```python
from build123d import *

# Parameters (mm, degrees)
SKETCH1_W                     = 104.5
SKETCH1_H                     = 59.5
BOSS_EXTRUDE1_DEPTH           = 73.36
CBORE_FOR_M4_SHCS2_AT_2_COUNT = 2
CBORE_FOR_M4_SHCS2_AT_2_PITCH = 73
CBORE_FOR_M4_SHCS2_AT_3_COUNT = 2
CBORE_FOR_M4_SHCS2_AT_3_PITCH = 83.725742756
CBORE_FOR_M4_SHCS2_AT_4_COUNT = 2
CBORE_FOR_M4_SHCS2_AT_4_PITCH = 41


with BuildPart() as part:
    # Sketch1 → Boss-Extrude1 (new body)
    with BuildSketch(Plane(origin=(0, 0, 0), x_dir=(1, 0, 0), z_dir=(0, 1, 0))):
        Rectangle(SKETCH1_W, SKETCH1_H)
    extrude(amount=BOSS_EXTRUDE1_DEPTH)

    # Sketch3 → CBORE for M4 SHCS2 (revolve, cut)
    with BuildSketch(Plane(origin=(-36.5, 0, 20.5), x_dir=(0, 0, -1), z_dir=(1, 0, 0))):
        Polygon((0, 0), (0, 73.36), (2.4, 73.36), (2.4, 59), (4, 59), (4, 0.025), (4.025, 0), align=None)
    cbore_for_m4_shcs2 = revolve(axis=Axis((-36.5, -6.35, 20.5), (0, 1, 0)), mode=Mode.SUBTRACT)

    # CBORE for M4 SHCS2 at 2: CBORE for M4 SHCS2 ×2
    with Locations(*[(i * CBORE_FOR_M4_SHCS2_AT_2_PITCH, 0, 0) for i in range(1, CBORE_FOR_M4_SHCS2_AT_2_COUNT)]):
        add(cbore_for_m4_shcs2, mode=Mode.SUBTRACT)

    # CBORE for M4 SHCS2 at 3: CBORE for M4 SHCS2 ×2
    with Locations(*[Vector(0.8718943254163863, 0, -0.48969407317906627) * (i * CBORE_FOR_M4_SHCS2_AT_3_PITCH) for i in range(1, CBORE_FOR_M4_SHCS2_AT_3_COUNT)]):
        add(cbore_for_m4_shcs2, mode=Mode.SUBTRACT)

    # CBORE for M4 SHCS2 at 4: CBORE for M4 SHCS2 ×2
    with Locations(*[(0, 0, -i * CBORE_FOR_M4_SHCS2_AT_4_PITCH) for i in range(1, CBORE_FOR_M4_SHCS2_AT_4_COUNT)]):
        add(cbore_for_m4_shcs2, mode=Mode.SUBTRACT)


solid = part.part
```
Design review of the part built by this model. Coordinates are the model's own, in mm. A direction names the side the tool comes from. Coordinates: 2 decimals unless noted, no trailing zeros. Order: outer loops, then holes, each group sorted by start corner. A loop starts at its lowest first (then second) coordinate and runs counter-clockwise, first axis right, second up.
1) Take a section at A-A, the plane x = -36.5. Give the boundary of the cut face in (y, z) (3 decimals).
2) Wall thickness on line 1 along Z through (x, y) = (-36.5, 69); line 2 along X through (y, z) = (68.75, -20.5); line 3 along X through (y, z) = (14, 20.5): over which ranges is each line inside the solid? List them lowest first.
3) Clearance check with a flat-ended pin moving along its axis: pin 1 (5.5 mm diameter, centred on x = -36.5, z = 20.5, fed in from -Y). State where the tip first meets the part, or that it passes through.
4) For faces 4 (the flat face through (-36.6, 59, -17.9)), 5 (the cylindrical face through (38.63, 66.08, 19.39)), list the 3-axis set-ups (+Z, -Z, +X, -X, +Y, -Y) from which the entire face can be reached by the end or side of a thin tool; tool diameter is ignored.
5) Take a section at C-C, the plane y = 50.5. Give the boundary of the cut face in (x, z).
6) Take a section at B-B, the plane z = 20.5. Give the boundary of the cut face in (x, y) (3 decimals), and give its area (3 significant figures).
7) Mouldability with a two-part tool opening along X and no side actions: class faces 1 (the flat face through (52.25, 36, 0)), 2 (the cylindrical face through (-40.466, 29.1, 21.021)), 3 (the flat face through (-52.25, 36, 0)) as +X half, -X half, draft (parallel to the pull), parting line (faces both ways), or undercut.
Returned:
1. outline: (0, -29.75) - (73.36, -29.75) - (73.36, -22.9) - (59, -22.9) - (59, -24.5) - (0.025, -24.5) - (0, -24.525) - close; (0, -16.475) - (0.025, -16.5) - (59, -16.5) - (59, -18.1) - (73.36, -18.1) - (73.36, 18.1) - (59, 18.1) - (59, 16.5) - (0.025, 16.5) - (0, 16.475) - close; (0, 24.525) - (0.025, 24.5) - (59, 24.5) - (59, 22.9) - (73.36, 22.9) - (73.36, 29.75) - (0, 29.75) - close
2. line 1: z = -29.75 to -22.9, -18.1 to 18.1, 22.9 to 29.75
2. line 2: x = -52.25 to -38.9, -34.1 to 34.1, 38.9 to 52.25
2. line 3: x = -52.25 to -40.5, -32.5 to 32.5, 40.5 to 52.25
3. pin 1: stops at y = 59
4. face 4: -Y
4. face 5: +Y, -Y
5. outline: (-52.25, -29.75) - (52.25, -29.75) - (52.25, 29.75) - (-52.25, 29.75) - close; hole circle Ø8 at (-36.5, -20.5); hole circle Ø8 at (-36.5, 20.5); hole circle Ø8 at (36.5, -20.5); hole circle Ø8 at (36.5, 20.5)
6. outline: (-52.25, 0) - (-40.525, 0) - (-40.5, 0.025) - (-40.5, 59) - (-38.9, 59) - (-38.9, 73.36) - (-52.25, 73.36) - close; (-34.1, 59) - (-32.5, 59) - (-32.5, 0.025) - (-32.475, 0) - (32.475, 0) - (32.5, 0.025) - (32.5, 59) - (34.1, 59) - (34.1, 73.36) - (-34.1, 73.36) - close; (38.9, 59) - (40.5, 59) - (40.5, 0.025) - (40.525, 0) - (52.25, 0) - (52.25, 73.36) - (38.9, 73.36) - close
6. area: 6,580 mm2
7. face 1: +X half
7. face 2: undercut
7. face 3: -X half
